Design review of the part built by this model. Coordinates are the model's own, in mm. Give positions to 0.01 mm unless a question says otherwise; leave off trailing zeros. Loops run counter-clockwise (first coordinate to the right, second up) from the corner with the lowest first, then second, coordinate; pieces in that order, holes last. Notation, with made-up numbers: (-5, 23) - (25, 23) arc R32 cw to (25, 50) - close; hole circle Ø6 at (-37, -13.5). An arc over 180 degrees is marked (long way). Write each question's results on one line, items separated by ' | '.
Autodesk Inventor part; units mm, degrees
ref_plane "Arbeitsebene1" through (44.5, 0, 0) normal (1, 0, 0) x (0, 1, 0)
ref_plane "XZ Plane" through (0, 0, 0) normal (0, 1, 0) x (-1, 0, 0)
ref_plane "XY Plane" through (0, 0, 0) normal (0, 0, 1) x (1, 0, 0)
sketch "Skizze1" plane through (0, 0, 0) normal (0, 1, 0) x (-1, 0, 0)
  line L0 (0, 0) -> (-89, 0)
  line L1 (-89, 0) -> (-89, 58)
  line L2 (-89, 58) -> (0, 58)
  line L3 (0, 58) -> (0, 0)
  dimension "d0" = 58
  dimension "d1" = 89
extrude "Extrusion1" add sketch "Skizze1" along normal blind 4
sketch "Skizze2" plane through (0, 4, 0) normal (0, 1, 0) x (1, 0, 0)
  line L0 (89, 0) -> (0, 0)
  line L1 (89, -58) -> (89, 0)
  line L2 (0, 0) -> (0, -58)
  line L3 (0, -58) -> (89, -58)
  point P0 (84, -6)
  point P1 (84, -52)
  point P2 (84, -40)
  point P3 (84, -18)
  point P4 (89, -29)
  point P5 (89, -29)
  dimension "d5" = 5
  dimension "d12" = 6
  dimension "d13" = 6
  dimension "d17" = 11
  dimension "d18" = 11
hole "Bohrung1" at (84, 4, 6) at (84, 4, 52) at (84, 4, 40) at (84, 4, 18) direction (0, -1, 0) diameter 4 depth 4
ref_plane "Arbeitsebene1" through (44.5, 0, 0) normal (1, 0, 0) x (0, 1, 0)
mirror "Spiegeln1" about plane through (44.5, 0, 0) normal (1, 0, 0) of "Bohrung1"
sketch "Skizze3" plane through (0, 4, 0) normal (0, 1, 0) x (1, 0, 0)
  line L0 (0, -58) -> (89, -58)
  circle A0 centre (84, -6) radius 2
  line L1 (89, 0) -> (0, 0)
  point P0 (64.5, -6)
  point P1 (24.5, -6)
  point P2 (44.5, -6)
  point P3 (44.5, -58)
  point P4 (64.5, -52)
  point P5 (44.5, -52)
  point P6 (24.5, -52)
  dimension "d27" = 20
  dimension "d28" = 20
  dimension "d44" = 6
  dimension "d45" = 6
hole "Bohrung2" at (64.5, 4, 6) at (24.5, 4, 6) at (44.5, 4, 6) at (64.5, 4, 52) at (44.5, 4, 52) at (24.5, 4, 52) direction (0, -1, 0) diameter 4 depth 4
sketch "Skizze4" plane through (0, 0, 0) normal (0, -1, 0) x (1, 0, 0)
  line L0 (0, 0) -> (0, 58)
  circle A0 centre (5, 52) radius 2
  circle A1 centre (84, 52) radius 2
  point P0 (5, 29)
  point P1 (84, 29)
  point P2 (0, 29)
hole "Bohrung3" at (5, 0, 29) at (84, 0, 29) direction (0, 1, 0) diameter 4 end through all
sketch "Sketch9" plane through (0, 0, 0) normal (0, -1, 0) x (1, 0, 0)
  line L0 (0, 0) -> (0, 58)
  line L1 (0, 58) -> (89, 58)
  point P0 (33.5, 29)
  point P1 (55.5, 29)
  point P2 (0, 29)
  point P3 (44.5, 58)
  dimension "d67" = 22
  dimension "d68" = 11
hole "Hole4" at (55.5, 0, 29) at (33.5, 0, 29) direction (0, 1, 0) diameter 4 depth 4
properties part number "1152" material "Kupfer"
(1) Take a section at C-C on z = 18. Give the boundary of the cut face in (x, y).
Answers below:
outline: (0, 0) - (3, 0) - (3, 4) - (0, 4) - close; (7, 0) - (82, 0) - (82, 4) - (7, 4) - close; (86, 0) - (89, 0) - (89, 4) - (86, 4) - close
(2) Take a section at D-D on y = 3.2. Count the separate pieces of the cut face and the enclosed holes in it, plus the area to 3 significant figures.
Answers below:
separate pieces: 1 | enclosed holes: 18 | area: 4,940 mm2
(3) Draft analysis for pull direction Z (two halves, no side actions). For faces 1 (the flat face through (44, 2, 0)), 2 (the flat face through (89, 2, 29)), 3 (the cylindrical face through (5, 2, 38)), state which applies: pulls with the +Z half, pulls with the -Z half, needs draft (parallel to the pull), parting line crosses it, or undercut.
Answers below:
face 1: pulls with the -Z half | face 2: needs draft | face 3: undercut
(4) Take a section at A-A on z = 29. Give the boundary of the cut face in (x, y), plus the area to 3 significant figures.
Answers below:
outline: (0, 0) - (3, 0) - (3, 4) - (0, 4) - close; (7, 0) - (31.5, 0) - (31.5, 4) - (7, 4) - close; (35.5, 0) - (53.5, 0) - (53.5, 4) - (35.5, 4) - close; (57.5, 0) - (82, 0) - (82, 4) - (57.5, 4) - close; (86, 0) - (89, 0) - (89, 4) - (86, 4) - close | area: 292 mm2
(5) Take a section at B-B on x = 55.5. Give the boundary of the cut face in (y, z), plus the area to 3 significant figures.
Answers below:
outline: (0, 0) - (4, 0) - (4, 27) - (0, 27) - close; (0, 31) - (4, 31) - (4, 58) - (0, 58) - close | area: 216 mm2
(6) Wall thickness on line 1 along X through (y, z) = (1.35, 6); line 2 along X through (y, z) = (1.4, 40); line 3 along Z through (x, y) = (64.5, 1.9): over which ranges is each line inside the solid? List them lowest first. Write a range as from..to.
Answers below:
line 1: 0..3, 7..22.5, 26.5..42.5, 46.5..62.5, 66.5..82, 86..89 | line 2: 0..3, 7..82, 86..89 | line 3: 0..4, 8..50, 54..58
